For this review, take the finished solid that the model builds, in its own axes (mm). Give positions to 0.01 mm unless a question says otherwise; leave off trailing zeros. Order: outer loops, then holes, each group sorted by start corner. A loop starts at its lowest first (then second) coordinate and runs counter-clockwise, first axis right, second up. Notation, with made-up numbers: M -16,-12 L 6,-12 A25 cw 6,1 Z; hole C -13.75,70 d6. An arc over 180 degrees is marked long. Answer as CSV lines item,"result". Start each with the question number.
1. We need section C-C, the plane z = 2.35. Give the boundary of the cut face in (x, y).
2. We need section B-B, the plane x = 0. Give the boundary of the cut face in (y, z), and give its area (3 significant figures).
3. Mouldability with a two-part tool opening along Y and no side actions: class faces 1 (the flat face through (-1, 1, 0)), 2 (the cylindrical face through (-0.98, -39.39, 1.48)) as pulls with the +Y half, pulls with the -Y half, needs draft (parallel to the pull), parting line crosses it, or undercut.
4. For line 1 along Y through (x, z) = (0, 1.1); line 2 along Y through (x, z) = (1, 2.85); line 3 along X through (y, z) = (40, 0.2), list the stretches that pass through material, from the lowest coordinate up.
5. Clearance check with flat-ended pins moving along their axes: P1, Ø1.5, axis at y = -32.5, z = 0.5, coming from the +X side; P2, Ø0.9, axis at x = -82, z = 1.5, coming from the -Y side; P3, Ø1.5, axis at x = -54.5, z = 1, coming from the +Y side. State where each tip first meets the part, or that it passes through.
6. We need section D-D, the plane y = 33. Give the boundary of the cut face in (x, z).
7. We need section A-A, the plane x = -40. Give the boundary of the cut face in (y, z), and give its area (3 significant figures).
from build123d import *

# Parameters (mm, degrees)
SKETCH_1_R      = 4.5
EXTRUDE_1_DEPTH = 3


with BuildPart() as part:
    # Эскиз1 → Бобышка-Вытянуть1 (new body)
    with BuildSketch(Plane.XY):
        Polygon((23, -23), (105, -23), (105, 23), (23, 23), (23, 50), (-23, 50), (-23, 23), (-105, 23), (-105, -23), (-23, -23), (-23, -50), (23, -50), align=None)
        with Locations((0, 35)):
            Circle(SKETCH_1_R, mode=Mode.SUBTRACT)
        with Locations((0, -35)):
            Circle(SKETCH_1_R, mode=Mode.SUBTRACT)
        with Locations((-90, 0)):
            Circle(SKETCH_1_R, mode=Mode.SUBTRACT)
        with Locations((-40, 0)):
            Circle(SKETCH_1_R, mode=Mode.SUBTRACT)
        with Locations(Location((40, 0, 0), (0, 0, 180))):  # turned: the seam where the file's is
            Circle(SKETCH_1_R, mode=Mode.SUBTRACT)
        with Locations(Location((90, 0, 0), (0, 0, 180))):  # turned: the seam where the file's is
            Circle(SKETCH_1_R, mode=Mode.SUBTRACT)
    extrude(amount=EXTRUDE_1_DEPTH)


solid = part.part
Result set:
1,outline,"M -105,-23 L -23,-23 L -23,-50 L 23,-50 L 23,-23 L 105,-23 L 105,23 L 23,23 L 23,50 L -23,50 L -23,23 L -105,23 Z; hole C -90,0 d9; hole C -40,0 d9; hole C 0,-35 d9; hole C 0,35 d9; hole C 40,0 d9; hole C 90,0 d9"
2,outline,"M -50,0 L -39.5,0 L -39.5,3 L -50,3 Z; M -30.5,0 L 30.5,0 L 30.5,3 L -30.5,3 Z; M 39.5,0 L 50,0 L 50,3 L 39.5,3 Z"
2,area,"246 mm2"
3,face 1,"needs draft"
3,face 2,"undercut"
4,line 1,"-50 to -39.5, -30.5 to 30.5, 39.5 to 50"
4,line 2,"-50 to -39.39, -30.61 to 30.61, 39.39 to 50"
4,line 3,"-23 to 23"
5,P1,"x = 23"
5,P2,"y = -23"
5,P3,"y = 23"
6,outline,"M -23,0 L -4.03,0 L -4.03,3 L -23,3 Z; M 4.03,0 L 23,0 L 23,3 L 4.03,3 Z"
7,outline,"M -23,0 L -4.5,0 L -4.5,3 L -23,3 Z; M 4.5,0 L 23,0 L 23,3 L 4.5,3 Z"
7,area,"111 mm2"
